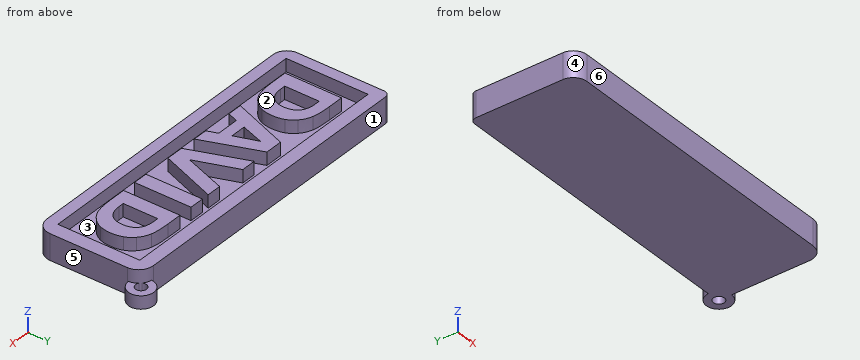
```python
from build123d import *

# Parameters (mm, degrees)
SKETCH002_R      = 2.929284
SKETCH002_R_2    = 1.279954
PAD002_DEPTH     = 3
PATH4830_W       = 13.200666
PATH4830_H       = 3.404056
EXTRUDE005_DEPTH = 3
EXTRUDE006_DEPTH = 3
EXTRUDE007_DEPTH = 3
EXTRUDE003_DEPTH = 3
EXTRUDE002_DEPTH = 3
EXTRUDE_DEPTH    = 3
EXTRUDE001_DEPTH = 3
EXTRUDE004_DEPTH = 3
SKETCH_W         = 68.637524
SKETCH_H         = 19.139309
PAD_DEPTH        = 3
PAD001_DEPTH     = 6


with BuildPart() as obj1:
    # Sketch002 → Pad002 (new body)
    with BuildSketch(Plane.XY):
        with Locations((37.034641, 12.51759)):
            Circle(SKETCH002_R)
        with Locations((37.034641, 12.51759)):
            Circle(SKETCH002_R_2, mode=Mode.SUBTRACT)
    extrude(amount=PAD002_DEPTH)


with BuildPart() as extrude005:
    # path4830 → Extrude005 (new body)
    with BuildSketch(Plane(origin=(12.588005, -0.084494, 0), x_dir=(0, -1, 0), z_dir=(0, 0, -1))):
        Rectangle(PATH4830_W, PATH4830_H)
    extrude(amount=-EXTRUDE005_DEPTH)


with BuildPart() as d2_corte:
    # path4832 → Extrude006 (new body)
    with BuildSketch(Plane(origin=(23.76392, -0.084496, 0), x_dir=(0, 1, 0), z_dir=(0, 0, 1))):
        with BuildLine():
            Line((4.027397, 2.754193), (-4.027397, 2.754193))
            Line((-4.027397, 2.754193), (-4.027397, 1.534037))
            add(Edge.make_bspline(
                [(-4.027397, 1.534037), (-4.027397, -0.552604), (-2.992918, -1.64898)],
                knots=[0, 0, 0, 1, 1, 1], degree=2))
            add(Edge.make_bspline(
                [(-2.992918, -1.64898), (-1.958435, -2.754193), (0.013263, -2.754193)],
                knots=[0, 0, 0, 1, 1, 1], degree=2))
            add(Edge.make_bspline(
                [(0.013263, -2.754193), (1.976123, -2.754193), (3.00176, -1.657821)],
                knots=[0, 0, 0, 1, 1, 1], degree=2))
            add(Edge.make_bspline(
                [(3.00176, -1.657821), (4.027397, -0.561446), (4.027397, 1.534037)],
                knots=[0, 0, 0, 1, 1, 1], degree=2))
            Line((4.027397, 1.534037), (4.027397, 2.754193))
        make_face()
    extrude(amount=EXTRUDE006_DEPTH)


with BuildPart() as d2:
    # path4832001 → Extrude007 (new body)
    with BuildSketch(Plane(origin=(23.816969, -0.084494, 0), x_dir=(0, -1, 0), z_dir=(0, 0, -1))):
        with BuildLine():
            Line((-6.600333, 6.211297), (-6.600333, 2.621564))
            add(Edge.make_bspline(
                [(-6.600333, 2.621564), (-6.600333, -0.384617), (-6.167086, -1.852338)],
                knots=[0, 0, 0, 1, 1, 1], degree=2))
            add(Edge.make_bspline(
                [(-6.167086, -1.852338), (-5.742686, -3.328901), (-4.717049, -4.381068)],
                knots=[0, 0, 0, 1, 1, 1], degree=2))
            add(Edge.make_bspline(
                [(-4.717049, -4.381068), (-3.824034, -5.309445), (-2.656929, -5.760371)],
                knots=[0, 0, 0, 1, 1, 1], degree=2))
            add(Edge.make_bspline(
                [(-2.656929, -5.760371), (-1.489823, -6.211297), (-0.013261, -6.211297)],
                knots=[0, 0, 0, 1, 1, 1], degree=2))
            add(Edge.make_bspline(
                [(-0.013261, -6.211297), (1.480986, -6.211297), (2.656933, -5.760371)],
                knots=[0, 0, 0, 1, 1, 1], degree=2))
            add(Edge.make_bspline(
                [(2.656933, -5.760371), (3.824038, -5.309445), (4.717053, -4.381068)],
                knots=[0, 0, 0, 1, 1, 1], degree=2))
            add(Edge.make_bspline(
                [(4.717053, -4.381068), (5.74269, -3.320059), (6.175932, -1.834655)],
                knots=[0, 0, 0, 1, 1, 1], degree=2))
            add(Edge.make_bspline(
                [(6.175932, -1.834655), (6.600333, -0.34925), (6.600333, 2.621564)],
                knots=[0, 0, 0, 1, 1, 1], degree=2))
            Line((6.600333, 2.621564), (6.600333, 6.211297))
            Line((6.600333, 6.211297), (-6.600333, 6.211297))
        make_face()
    extrude(amount=-EXTRUDE007_DEPTH)

    # Cut001: cut D2-Corte
    add(d2_corte.part, mode=Mode.SUBTRACT)


with BuildPart() as a_corte:
    # path4826001 → Extrude003 (new body)
    with BuildSketch(Plane(origin=(-10.577261, 0.795254, 0), x_dir=(0, 1, 0), z_dir=(0, 0, 1))):
        Polygon((-2.625987, 1.808129), (-2.625987, -1.808129), (2.625987, -0.004421), align=None)
    extrude(amount=EXTRUDE003_DEPTH)


with BuildPart() as a:
    # path4826 → Extrude002 (new body)
    with BuildSketch(Plane(origin=(-10.577261, -0.084494, 0), x_dir=(0, -1, 0), z_dir=(0, 0, -1))):
        Polygon((4.195393, -2.665773), (4.195393, 2.656935), (6.600333, 3.496895), (6.600333, 6.918635), (-6.600333, 2.029174), (-6.600333, -2.029169), (6.600333, -6.918635), (6.600333, -3.496895), align=None)
    extrude(amount=-EXTRUDE002_DEPTH)

    # Cut: cut A-Corte
    add(a_corte.part, mode=Mode.SUBTRACT)


with BuildPart() as d1_corte:
    # path4824 → Extrude (new body)
    with BuildSketch(Plane(origin=(-24.794724, -0.084496, 0), x_dir=(0, 1, 0), z_dir=(0, 0, 1))):
        with BuildLine():
            Line((4.027397, 2.754193), (-4.027397, 2.754193))
            Line((-4.027397, 2.754193), (-4.027397, 1.534037))
            add(Edge.make_bspline(
                [(-4.027397, 1.534037), (-4.027397, -0.552609), (-2.992918, -1.64898)],
                knots=[0, 0, 0, 1, 1, 1], degree=2))
            add(Edge.make_bspline(
                [(-2.992918, -1.64898), (-1.958435, -2.754193), (0.013263, -2.754193)],
                knots=[0, 0, 0, 1, 1, 1], degree=2))
            add(Edge.make_bspline(
                [(0.013263, -2.754193), (1.976123, -2.754193), (3.00176, -1.657821)],
                knots=[0, 0, 0, 1, 1, 1], degree=2))
            add(Edge.make_bspline(
                [(3.00176, -1.657821), (4.027397, -0.56145), (4.027397, 1.534037)],
                knots=[0, 0, 0, 1, 1, 1], degree=2))
            Line((4.027397, 1.534037), (4.027397, 2.754193))
        make_face()
    extrude(amount=EXTRUDE_DEPTH)


with BuildPart() as d1:
    # path4824001 → Extrude001 (new body)
    with BuildSketch(Plane(origin=(-24.741674, -0.084494, 0), x_dir=(0, -1, 0), z_dir=(0, 0, -1))):
        with BuildLine():
            Line((-6.600333, 6.211299), (-6.600333, 2.621566))
            add(Edge.make_bspline(
                [(-6.600333, 2.621566), (-6.600333, -0.384615), (-6.167086, -1.852336)],
                knots=[0, 0, 0, 1, 1, 1], degree=2))
            add(Edge.make_bspline(
                [(-6.167086, -1.852336), (-5.742686, -3.328903), (-4.717049, -4.381066)],
                knots=[0, 0, 0, 1, 1, 1], degree=2))
            add(Edge.make_bspline(
                [(-4.717049, -4.381066), (-3.824034, -5.309443), (-2.656929, -5.760369)],
                knots=[0, 0, 0, 1, 1, 1], degree=2))
            add(Edge.make_bspline(
                [(-2.656929, -5.760369), (-1.489823, -6.211299), (-0.013261, -6.211299)],
                knots=[0, 0, 0, 1, 1, 1], degree=2))
            add(Edge.make_bspline(
                [(-0.013261, -6.211299), (1.480986, -6.211299), (2.656933, -5.760369)],
                knots=[0, 0, 0, 1, 1, 1], degree=2))
            add(Edge.make_bspline(
                [(2.656933, -5.760369), (3.824038, -5.309443), (4.717053, -4.381066)],
                knots=[0, 0, 0, 1, 1, 1], degree=2))
            add(Edge.make_bspline(
                [(4.717053, -4.381066), (5.74269, -3.320062), (6.175932, -1.834653)],
                knots=[0, 0, 0, 1, 1, 1], degree=2))
            add(Edge.make_bspline(
                [(6.175932, -1.834653), (6.600333, -0.349248), (6.600333, 2.621566)],
                knots=[0, 0, 0, 1, 1, 1], degree=2))
            Line((6.600333, 2.621566), (6.600333, 6.211299))
            Line((6.600333, 6.211299), (-6.600333, 6.211299))
        make_face()
    extrude(amount=-EXTRUDE001_DEPTH)

    # Cut002: cut D1-Corte
    add(d1_corte.part, mode=Mode.SUBTRACT)


with BuildPart() as obj2:
    # path4828 → Extrude004 (new body)
    with BuildSketch(Plane(origin=(2.207842, -0.084494, 0), x_dir=(0, -1, 0), z_dir=(0, 0, -1))):
        Polygon((-6.600333, 6.918635), (-6.600333, 3.496895), (3.143226, -0.004421), (-6.600333, -3.496895), (-6.600333, -6.918635), (6.600333, -2.029169), (6.600333, 2.029169), align=None)
    extrude(amount=-EXTRUDE004_DEPTH)

    # Fusion: union Extrude005, D2, A, D1
    add(extrude005.part)
    add(d2.part)
    add(a.part)
    add(d1.part)


with BuildPart() as obj2_1:
    # Fusion placement: moved
    add(obj2.part.moved(Location((0, 0, 3))))


with BuildPart() as corte_base:
    # Sketch → Pad (new body)
    with BuildSketch(Plane.XY.offset(3)):
        with Locations((-0.549982, 0.109995)):
            Rectangle(SKETCH_W, SKETCH_H)
    extrude(amount=PAD_DEPTH)


with BuildPart() as obj3:
    # Sketch001 → Pad001 (new body)
    with BuildSketch(Plane.XY):
        with BuildLine():
            Line((-36.122698, 12.741634), (33.658366, 12.741634))
            ThreePointArc((37.068661, 9.33134), (36.069809, 11.742782), (33.658366, 12.741634))
            Line((37.068661, 9.33134), (37.068661, -8.689686))
            ThreePointArc((33.627401, -12.130946), (36.060739, -11.123024), (37.068661, -8.689686))
            Line((33.627401, -12.130946), (-34.409048, -12.130946))
            ThreePointArc((-37.57005, -8.969945), (-36.644214, -11.20511), (-34.409048, -12.130946))
            Line((-37.57005, -8.969945), (-37.57005, 11.294283))
            ThreePointArc((-36.122698, 12.741634), (-37.14613, 12.317715), (-37.57005, 11.294283))
        make_face()
    extrude(amount=PAD001_DEPTH)

    # Cut003: cut Corte-Base
    add(corte_base.part, mode=Mode.SUBTRACT)

    # Fusion001: union obj2
    add(obj2_1.part)

    # Fusion002: union obj1
    add(obj1.part)


solid = obj3.part
```
Could you check a few things on this model? Use its own coordinates, in mm. Face numbers are marked on the shaded views. A direction names the side the tool comes from. Give positions to 0.01 mm unless a question says otherwise; leave off trailing zeros. Order: outer loops, then holes, each group sorted by start corner. A loop starts at its lowest first (then second) coordinate and runs counter-clockwise, first axis right, second up.
Q1. I'm going to push flat-ended pins straight in: P1, Ø10, axis at x = 11.5, y = -2.5, coming from the -Z side; P2, Ø3.5, axis at y = -1.5, z = 4, coming from the +X side; P3, Ø2.5, axis at x = -11, z = 5, coming from the +Y side. Where does each tip first touch, or does it pass through?
Q2. Suppose I cut it at C-C, the plane z = 0.75. Write out the boundary of the cut face in (x, y).
Q3. For the marked faces 1 and 2, which set-ups out of +Z, -Z, +X, -X, +Y, -Y let a thin tool reach every point of the face, with its end or its side?
Q4. Suppose I cut it at A-A, the plane z = 4.25. Count the separate pieces of the cut face and the enclosed holes in it, and give its area (3 significant figures).
Q5. We'd pull the mould along X, two halves only. Please class the marked faces 3, 4, 5 and 6: +X half, -X half, draft (parallel to the pull), parting line (faces both ways), or undercut.
Q6. Suppose I cut it at B-B, the plane x = -2. Write out the boundary of the cut face in (y, z), and give its area (3 significant figures).
Q7. If I drill on line 1 along Y through (x, z) = (22, 4.75); line 2 along Y through (x, z) = (-29, 5.25); line 3 along Y through (x, z) = (25, 5.5), over which ranges is the centre line in solid material (lowest first)?
Solution:
1. P1: stops at z = 0
1. P2: stops at x = 37.07
1. P3: stops at y = 12.74
2. outline: (-37.57, -8.97) arc R3.16 ccw to (-34.41, -12.13) - (33.63, -12.13) arc R3.44 ccw to (37.07, -8.69) - (37.07, 9.33) arc R3.41 ccw to (37.06, 9.59) arc R2.93 ccw (long way) to (34.11, 12.71) arc R3.41 ccw to (33.66, 12.74) - (-36.12, 12.74) arc R1.45 ccw to (-37.57, 11.29) - close; hole (35.93, 11.88) arc R3.41 cw to (36.33, 11.45) arc R1.28 ccw (long way) to start
3. face 1: +Z, -Z, -X, +Y
3. face 2: +Z, +X, -X, +Y, -Y
4. separate pieces: 6
4. enclosed holes: 4
4. area: 973 mm2
5. face 3: undercut
5. face 4: -X half
5. face 5: +X half
5. face 6: draft
6. outline: (-12.13, 0) - (12.74, 0) - (12.74, 6) - (9.68, 6) - (9.68, 3) - (6.52, 3) - (6.52, 6) - (-0.8, 6) - (-0.8, 3) - (-9.46, 3) - (-9.46, 6) - (-12.13, 6) - close
6. area: 114 mm2
7. line 1: y = -12.13 to -9.46, -6.68 to -4.11, 3.94 to 6.51, 9.68 to 12.74
7. line 2: y = -12.13 to -9.46, -6.68 to 6.52, 9.68 to 12.74
7. line 3: y = -12.13 to -9.46, -6.41 to -3.41, 3.25 to 6.24, 9.68 to 12.74
